Design review of the part built by this model. Coordinates are the model's own, in mm. Coordinates: 2 decimals unless noted, no trailing zeros. Write each loop counter-clockwise with the first axis right and the second up, starting at its lowest first coordinate (ties: lowest second). Pieces come first, ordered by that corner, then holes. Notation, with made-up numbers: (16.25, 21) -> (29.25, 21) arc R18 ccw to (29.25, 37) -> close; hole circle Ø8 at (1.25, 55). An arc over 180 degrees is marked (long way). Answer in a Markdown table with one row per item. Add a question column.
Item 1: Take a section at B-B, the plane y = -16.75. Write out the cut boundary in (x, z).
Item 2: Clearance check with flat-ended pins moving along their axes: P1, Ø1.5, axis at x = 13.5, z = 4.5, coming from the -Y side; P2, Ø5, axis at x = 10, y = -8, coming from the -Z side; P3, Ø4, axis at x = 4, z = 5.5, coming from the +Y side; P4, Ø2, axis at x = 6, z = 3.5, coming from the -Y side. State where each tip first meets the part, or that it passes through.
Item 3: Take a section at C-C, the plane z = 4.5. Write out the cut boundary in (x, y), and give its area (3 significant figures).
Item 4: To check wall thickness, follow line 1 (Y direction, x = 6, z = 5.75); line 2 (Y direction, x = 2.5, z = 1.75); line 3 (Z direction, x = 5, y = -15). State the ranges of each line that lie inside material, in increasing order.
from build123d import *

# Parameters (mm, degrees)
F0_W     = 12.7
F0_H     = 7.62
F1_DEPTH = 15.5956
F2_SIZE  = 7.61999


# Not quite as in the source:
# - a fillet or chamfer is up to 0.001 mm smaller than in the source, because OpenCascade refuses the exact size


with BuildPart() as f1:
    # F0 (on Right) → F1 (new body)
    with BuildSketch(Plane.YZ):
        with Locations((-6.35, 3.81)):
            Rectangle(F0_W, F0_H)
        Polygon((-20.7394696772, 5.931511987), (-12.7, 0), (-12.7, 7.62), align=None)
    extrude(amount=F1_DEPTH)

    # F2 (size 7.62 in the source; OpenCascade refuses exactly that, so slightly less here)
    f2_edges = [f1.edges().sort_by_distance(p)[0] for p in [
        (7.7978, 0, 7.62),
    ]]
    chamfer(f2_edges, length=F2_SIZE)


solid = f1.part
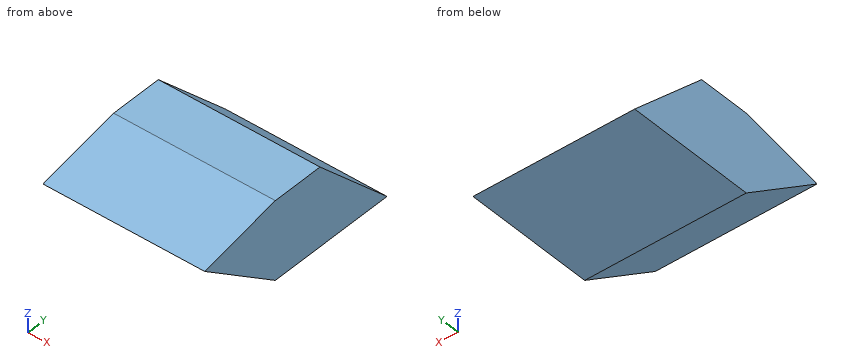
Answers:
| question | item | result |
|---|---|---|
| 1 | outline | (0, 2.99) -> (15.6, 2.99) -> (15.6, 6.77) -> (0, 6.77) -> close |
| 2 | P1 | stops at y = -19.82 |
| 2 | P2 | stops at z = 0 |
| 2 | P3 | stops at y = -3.5 |
| 2 | P4 | stops at y = -18.8 |
| 3 | outline | (0, -18.8) -> (15.6, -18.8) -> (15.6, -4.5) -> (0, -4.5) -> close |
| 3 | area | 223 mm^2 |
| 4 | line 1 | y = -20.49 to -5.75 |
| 4 | line 2 | y = -15.07 to -1.75 |
| 4 | line 3 | z = 1.7 to 7.14 |
